```python
from build123d import *

# Parameters (mm, degrees)
SKETCH1_R           = 22
BOSS_EXTRUDE1_DEPTH = 10
SKETCH3_R           = 10
BOSS_EXTRUDE2_DEPTH = 10
SKETCH4_R           = 2.6
BOSS_EXTRUDE3_DEPTH = 10
SKETCH7_W           = 10.354007758
SKETCH7_H           = 7.823019208
BOSS_EXTRUDE4_DEPTH = 10


with BuildPart() as part:
    # Sketch1 → Boss-Extrude1 (new body)
    with BuildSketch(Plane.XY):
        Circle(SKETCH1_R)
    extrude(amount=BOSS_EXTRUDE1_DEPTH)

    # Sketch3 → Boss-Extrude2 (add)
    with BuildSketch(Plane(origin=(0, 0, 0), x_dir=(-1, 0, 0), z_dir=(0, 0, -1))):
        Circle(SKETCH3_R)
    extrude(amount=BOSS_EXTRUDE2_DEPTH)

    # Sketch4 → Boss-Extrude3 (add)
    with BuildSketch(Plane(origin=(0, 0, 0), x_dir=(-1, 0, 0), z_dir=(0, 0, -1))):
        with Locations((17.1, 0)):
            Circle(SKETCH4_R)
        with Locations((-8.55, -14.809034405)):
            Circle(SKETCH4_R)
        with Locations((-8.55, 14.809034405)):
            Circle(SKETCH4_R)
    extrude(amount=BOSS_EXTRUDE3_DEPTH)

    # Sketch7 → Boss-Extrude4 (add)
    with BuildSketch(Plane(origin=(0, 0, -10), x_dir=(-1, 0, 0), z_dir=(0, 0, -1))):
        Rectangle(SKETCH7_W, SKETCH7_H)
    extrude(amount=BOSS_EXTRUDE4_DEPTH)


solid = part.part
```
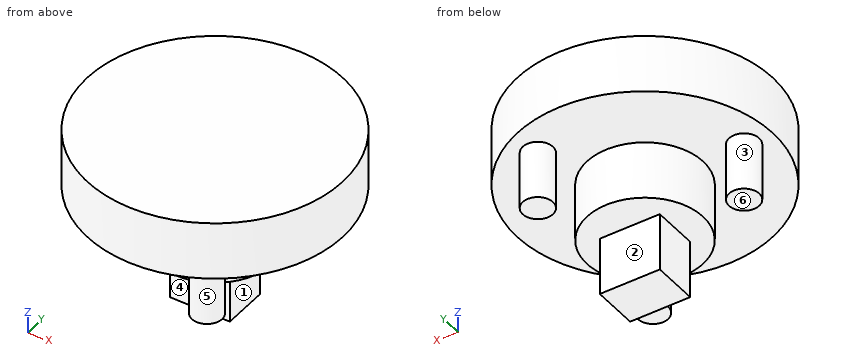
CAD build for the part. Positions are in the model's coordinates, mm. Face numbers are marked on the shaded views. A direction names the side the tool comes from. Round coordinates to 2 decimals unless told otherwise and drop trailing zeros. Loops run counter-clockwise (first coordinate to the right, second up) from the corner with the lowest first, then second, coordinate; pieces in that order, holes last. Notation, with made-up numbers: M 9.25,-15 L 45.25,-15 A17 ccw 45.25,4 Z; hole C 64,60 d10. An arc over 180 degrees is marked long. Return JSON: item names as keys, results as strings. Group by question number.
(1) Tool access for the marked faces 4, 5 and 6: list every direction of +Z, -Z, +X, -X, +Y, -Y with a clear straight run to the whole face (end or side of a thin tool).
(2) Saw through at C-C, the plane z = -15.25. List the corners of the cut face in (x, y).
(3) Wall check: probe 1 along Z at (x, y) = (2, 11); probe 2 along X at (y, z) = (-1.5, -10.25); probe 3 along Y at (x, z) = (5, -16). Give the ranges that are in metal, low to high. Write a range as [from, to].
(4) Drop flat-ended pins along their axis: P1, Ø1.5, axis at x = 3, y = -15, coming from the -Z side; P2, Ø3, axis at x = 5, z = -2, coming from the -Y side; P3, Ø5, axis at x = 3, z = -10.5, coming from the -Y side; P4, Ø10, axis at x = -1, y = 4.5, coming from the -Z side. Give the stop position or say it passes through.
(5) Saw through at B-B, the plane y = 0. List the corners of the cut face in (x, z), and give its area (3 significant figures).
(6) Mould opens along X. For the marked faces 1, 2 and 3 say: +X half, -X half, draft (parallel to the pull), parting line (faces both ways), or undercut.
(7) Saw through at A-A, the plane x = 0. List the corners of the cut face in (y, z), and give its area (3 significant figures).
(8) Saw through at D-D, the plane x = -17.1. List the corners of the cut face in (y, z), and give its area (3 significant figures).
Answer list:
{
 "1": {"face 4": "-Z, +X, -X, -Y", "face 5": "-Z", "face 6": "-Z, -X, +Y, -Y"},
 "2": {"outline": "M -5.18,-3.91 L 5.18,-3.91 L 5.18,3.91 L -5.18,3.91 Z"},
 "3": {"probe 1": "[0, 10]", "probe 2": "[-5.18, 5.18]", "probe 3": "[-3.91, 3.91]"},
 "4": {"P1": "z = 0", "P2": "y = -16.41", "P3": "y = -9.98", "P4": "z = -20"},
 "5": {"outline": "M -22,0 L -19.7,0 L -19.7,-10 L -14.5,-10 L -14.5,0 L -10,0 L -10,-10 L -5.18,-10 L -5.18,-20 L 5.18,-20 L 5.18,-10 L 10,-10 L 10,0 L 22,0 L 22,10 L -22,10 Z", "area": "796 mm2"},
 "6": {"face 1": "+X half", "face 2": "draft", "face 3": "undercut"},
 "7": {"outline": "M -22,0 L -10,0 L -10,-10 L -3.91,-10 L -3.91,-20 L 3.91,-20 L 3.91,-10 L 10,-10 L 10,0 L 22,0 L 22,10 L -22,10 Z", "area": "718 mm2"},
 "8": {"outline": "M -13.84,0 L -2.6,0 L -2.6,-10 L 2.6,-10 L 2.6,0 L 13.84,0 L 13.84,10 L -13.84,10 Z", "area": "329 mm2"}
}
